Here's how the part is built. I have some questions about the finished solid (model axes, mm). Face numbers are marked on the shaded views. Round coordinates to 2 decimals unless told otherwise and drop trailing zeros. Write each loop counter-clockwise with the first axis right and the second up, starting at its lowest first coordinate (ties: lowest second). Pieces come first, ordered by that corner, then holes. Notation, with made-up numbers: (20.25, -3.75) -> (65.25, -3.75) arc R23 cw to (65.25, 32.25) -> close; hole circle Ø10 at (72, 77.5). An arc over 180 degrees is marked (long way). Answer as CSV lines item,"result".
```python
from build123d import *

# Parameters (mm, degrees)
SKETCH1_R           = 6.5
SKETCH1_R_2         = 6
BOSS_EXTRUDE1_DEPTH = 10
BOSS_EXTRUDE2_START = -1
SKETCH2_R           = 8
SKETCH2_R_2         = 6
BOSS_EXTRUDE2_DEPTH = 1
LPATTERN1_COUNT     = 2
LPATTERN1_PITCH     = 9
FILLET1_R           = 1


with BuildPart() as part:
    # Sketch1 → Boss-Extrude1 (new body)
    with BuildSketch(Plane(origin=(0, 0, 0), x_dir=(1, 0, 0), z_dir=(0, 1, 0))):
        with Locations(Location((0, 0, 0), (0, 0, 270))):
            Circle(SKETCH1_R)
        with Locations(Location((0, 0, 0), (0, 0, 270))):
            Circle(SKETCH1_R_2, mode=Mode.SUBTRACT)
    extrude(amount=BOSS_EXTRUDE1_DEPTH)

    # Sketch2 → Boss-Extrude2 (add)
    with BuildSketch(Plane(origin=(0, 10, 0), x_dir=(1, 0, 0), z_dir=(0, 1, 0)).offset(BOSS_EXTRUDE2_START)):
        with Locations(Location((0, 0, 0), (0, 0, 270))):
            Circle(SKETCH2_R)
        with Locations(Location((0, 0, 0), (0, 0, 270))):
            Circle(SKETCH2_R_2, mode=Mode.SUBTRACT)
    boss_extrude2 = extrude(amount=BOSS_EXTRUDE2_DEPTH)

    # LPattern1: Boss-Extrude2 ×2
    with Locations(*[(0, -i * LPATTERN1_PITCH, 0) for i in range(1, LPATTERN1_COUNT)]):
        add(boss_extrude2)

    # Fillet1
    fillet1_edges = [part.edges().sort_by_distance(p)[0] for p in [
        (0, 9, -6.5),
        (0, 1, -6.5),
    ]]
    fillet(fillet1_edges, radius=FILLET1_R)


solid = part.part
```
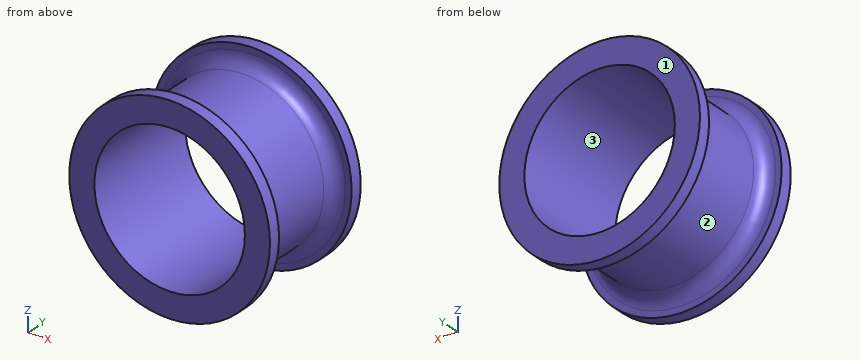
1. Suppose I cut it at A-A on x = 0. Please give me the cut outline in (y, z).
Numbers:
outline,"(0, -8) -> (1, -8) -> (1, -7.5) arc R1 cw to (2, -6.5) -> (8, -6.5) arc R1 cw to (9, -7.5) -> (9, -8) -> (10, -8) -> (10, -6) -> (0, -6) -> close; (0, 6) -> (10, 6) -> (10, 8) -> (9, 8) -> (9, 7.5) arc R1 cw to (8, 6.5) -> (2, 6.5) arc R1 cw to (1, 7.5) -> (1, 8) -> (0, 8) -> close"
2. For pin 1 Ø2 at (y, z) = (8.5, 4.5) entering from +X; pin 2 Ø4 at (y, z) = (3.5, 3) entering from +X; pin 3 Ø1 at (y, z) = (2.5, 4.5) entering from +X, each with a flat end and sliding along its axis, tell me the tip position at first contact or that it passes through.
Numbers:
pin 1,"stops at x = 7.13"
pin 2,"stops at x = 6.42"
pin 3,"stops at x = 5.12"
3. If we mould it in two halves opening along Z, with no side actions, what happens to the marked faces 1, 2 and 3? For each: released by +Z, released by -Z, zero draft, split by the parting line, or undercut.
Numbers:
face 1,"zero draft"
face 2,"split by the parting line"
face 3,"undercut"
4. Suppose I cut it at B-B on z = 0. Please give me the cut outline in (x, y).
Numbers:
outline,"(-8, 0) -> (-6, 0) -> (-6, 10) -> (-8, 10) -> (-8, 9) -> (-7.5, 9) arc R1 cw to (-6.5, 8) -> (-6.5, 2) arc R1 cw to (-7.5, 1) -> (-8, 1) -> close; (6, 0) -> (8, 0) -> (8, 1) -> (7.5, 1) arc R1 cw to (6.5, 2) -> (6.5, 8) arc R1 cw to (7.5, 9) -> (8, 9) -> (8, 10) -> (6, 10) -> close"
5. Suppose I cut it at C-C on y = 6. Please give me the cut outline in (x, z), and give its area (3 significant figures).
Numbers:
outline,"circle Ø13 at (0, 0); hole circle Ø12 at (0, 0)"
area,"19.6 mm^2"
6. If I drill on line 1 (X direction, y = 3.5, z = 0); line 2 (Z direction, x = 4.5, y = 6); line 3 (Z direction, x = 2, y = 0.75), over which ranges is the centre line in solid material (lowest first)?
Numbers:
line 1,"x = -6.5 to -6, 6 to 6.5"
line 2,"z = -4.69 to -3.97, 3.97 to 4.69"
line 3,"z = -7.75 to -5.66, 5.66 to 7.75"
7. Suppose I cut it at D-D on y = 1.25. Please give me the cut outline in (x, z), and give its area (3 significant figures).
Numbers:
outline,"circle Ø13.68 at (0, 0); hole circle Ø12 at (0, 0)"
area,"33.8 mm^2"
